Here's how the part is built. I have some questions about the finished solid (model axes, mm). Coordinates: 2 decimals unless noted, no trailing zeros. Order: outer loops, then holes, each group sorted by start corner. A loop starts at its lowest first (then second) coordinate and runs counter-clockwise, first axis right, second up. Notation, with made-up numbers: (49.25, -11) - (96.25, -11) arc R17 cw to (96.25, 16) - close; hole circle Ø4 at (64, -30). An arc over 180 degrees is marked (long way). Answer as CSV lines item,"result". Start each with the question number.
Item 1: I need wall thicknesses on line 1 (Y direction, x = -42.75, z = 1.35); line 2 (Y direction, x = -74, z = 1.5); line 3 (Z direction, x = -57, y = -1.5). Which ranges of each line are inside material? Lowest first, please.
Item 2: I'm going to push flat-ended pins straight in: pin 1 (11 mm diameter, centred on x = -2, y = -0.5, fed in from +Z); pin 2 (2 mm diameter, centred on x = -52.5, z = 0.5, fed in from +Y); pin 3 (1.4 mm diameter, centred on x = -50.5, z = 0.5, fed in from -Y); pin 4 (2.5 mm diameter, centred on x = -42.75, y = -5, fed in from +Z). Where does each tip first touch, or does it pass through?
Item 3: Imagine slicing it at C-C on x = 3. List the corners of the cut face in (y, z) for me, and give its area (3 significant figures).
Item 4: Imagine slicing it at A-A on x = -42.75. List the corners of the cut face in (y, z) for me.
Item 5: Imagine slicing it at B-B on y = -14.1. List the corners of the cut face in (x, z) for me, and give its area (3 significant figures).
Item 6: Imagine slicing it at D-D on y = -23.2. List the corners of the cut face in (x, z) for me, and give its area (3 significant figures).
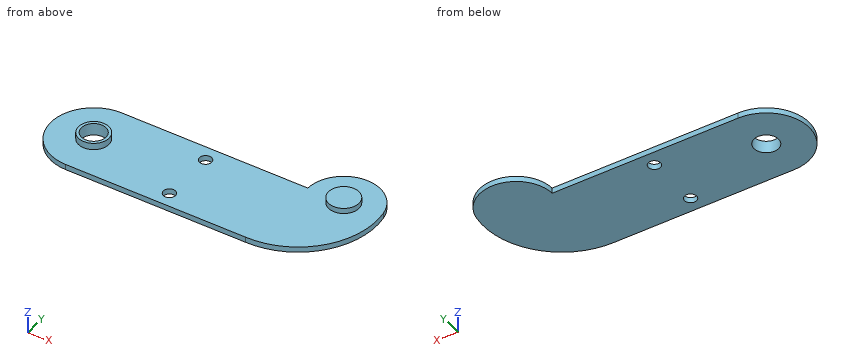
from build123d import *

# Parameters (mm, degrees)
ESBO_O1_R                = 4.05
ESBO_O1_R_2              = 2
RESSALTO_EXTRUS_O1_DEPTH = 1.8
ESBO_O2_R                = 5
RESSALTO_EXTRUS_O2_DEPTH = 3.6
ESBO_O4_R                = 5
ESBO_O4_R_2              = 4.05
RESSALTO_EXTRUS_O3_DEPTH = 2.2


with BuildPart() as part:
    # Esboço1 → Ressalto-extrusão1 (new body)
    with BuildSketch(Plane.XY):
        with BuildLine():
            Line((-12, 0), (-74, 0))
            ThreePointArc((-74, 0), (-88.1, -14.1), (-74, -28.2))
            Line((-74, -28.2), (-14, -28.2))
            ThreePointArc((-14, -28.2), (6.004940765, -19.140656488), (11.826301138, 2.034355278))
            ThreePointArc((11.826301138, 2.034355278), (-1.020878628, 11.956496428), (-12, 0))
        make_face()
        with Locations((-74, -14.1)):
            Circle(ESBO_O1_R, mode=Mode.SUBTRACT)
        with Locations((-42.75, -5)):
            Circle(ESBO_O1_R_2, mode=Mode.SUBTRACT)
        with Locations((-42.75, -23.2)):
            Circle(ESBO_O1_R_2, mode=Mode.SUBTRACT)
    extrude(amount=RESSALTO_EXTRUS_O1_DEPTH)

    # Esboço2 → Ressalto-extrusão2 (add)
    with BuildSketch(Plane.XY):
        with Locations(Location((0, 0, 0), (0, 0, 180))):
            Circle(ESBO_O2_R)
    extrude(amount=RESSALTO_EXTRUS_O2_DEPTH)

    # Esboço4 → Ressalto-extrusão3 (add)
    with BuildSketch(Plane.XY.offset(1.8)):
        with Locations(Location((-74, -14.1, 0), (0, 0, 180))):
            Circle(ESBO_O4_R)
        with Locations((-74, -14.1)):
            Circle(ESBO_O4_R_2, mode=Mode.SUBTRACT)
    extrude(amount=RESSALTO_EXTRUS_O3_DEPTH)


solid = part.part
Responses:
1,line 1,"y = -28.2 to -25.2, -21.2 to -7, -3 to 0"
1,line 2,"y = -28.2 to -18.15, -10.05 to 0"
1,line 3,"z = 0 to 1.8"
2,pin 1,"stops at z = 3.6"
2,pin 2,"stops at y = 0"
2,pin 3,"stops at y = -28.2"
2,pin 4,"passes through"
3,outline,"(-22.12, 0) - (11.62, 0) - (11.62, 1.8) - (4, 1.8) - (4, 3.6) - (-4, 3.6) - (-4, 1.8) - (-22.12, 1.8) - close"
3,area,"75.1 mm^2"
4,outline,"(-28.2, 0) - (-25.2, 0) - (-25.2, 1.8) - (-28.2, 1.8) - close; (-21.2, 0) - (-7, 0) - (-7, 1.8) - (-21.2, 1.8) - close; (-3, 0) - (0, 0) - (0, 1.8) - (-3, 1.8) - close"
5,outline,"(-88.1, 0) - (-78.05, 0) - (-78.05, 4) - (-79, 4) - (-79, 1.8) - (-88.1, 1.8) - close; (-69.95, 0) - (9.38, 0) - (9.38, 1.8) - (-69, 1.8) - (-69, 4) - (-69.95, 4) - close"
5,area,"165 mm^2"
6,outline,"(-84.77, 0) - (-44.75, 0) - (-44.75, 1.8) - (-84.77, 1.8) - close; (-40.75, 0) - (1.63, 0) - (1.63, 1.8) - (-40.75, 1.8) - close"
6,area,"148 mm^2"
